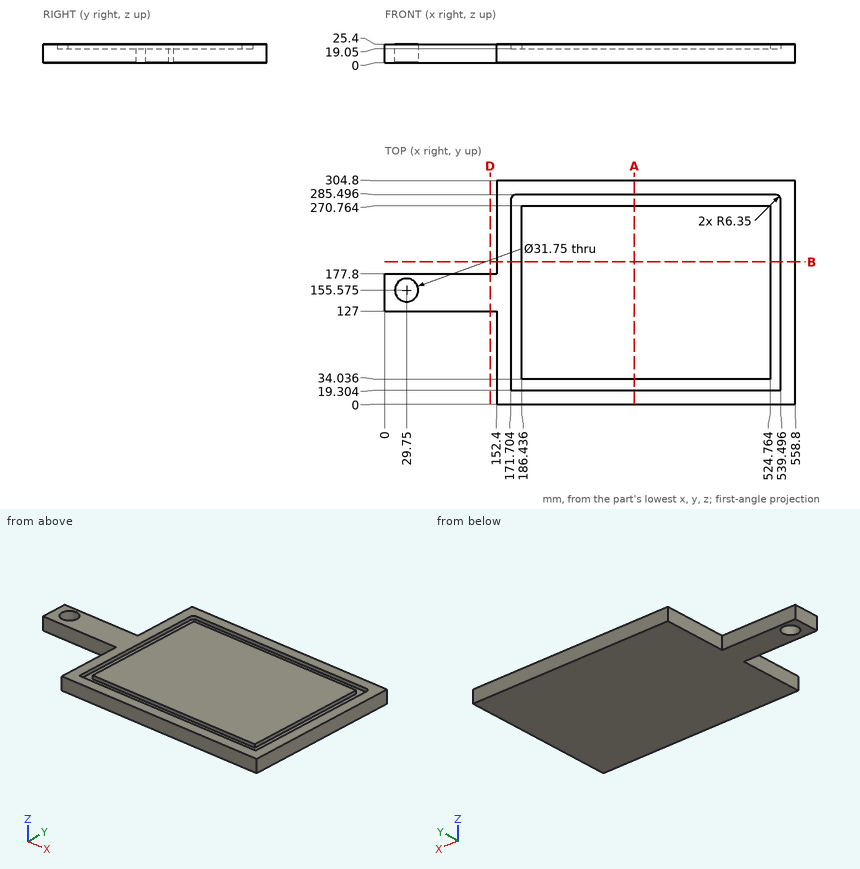
Geometry: see drawing. Coordinates: mm, zero at the bounding-box minimum. Coordinates: 2 decimals unless noted, no trailing zeros. Loops run counter-clockwise (first coordinate to the right, second up) from the corner with the lowest first, then second, coordinate; pieces in that order, holes last. Notation, with made-up numbers: (25.25, 65.5) - (76.25, 65.5) arc R26 cw to (76.25, 91.5) - close; hole circle Ø4 at (63, 47.25). An arc over 180 degrees is marked (long way). Return JSON: item names as keys, results as strings.
Q1. Section B-B, the plane y = 194. Return loops of the section in (x, z), plus the area to 3 significant figures.
Results:
{"outline": "(152.4, 0) - (558.8, 0) - (558.8, 25.4) - (539.5, 25.4) - (539.5, 19.05) - (524.76, 19.05) - (524.76, 25.4) - (186.44, 25.4) - (186.44, 19.05) - (171.7, 19.05) - (171.7, 25.4) - (152.4, 25.4) - close", "area": "10,100 mm2"}
Q2. Section A-A, the plane x = 340. Return loops of the section in (y, z).
Results:
{"outline": "(0, 0) - (304.8, 0) - (304.8, 25.4) - (285.5, 25.4) - (285.5, 19.05) - (270.76, 19.05) - (270.76, 25.4) - (34.04, 25.4) - (34.04, 19.05) - (19.3, 19.05) - (19.3, 25.4) - (0, 25.4) - close"}
Q3. Contact query for flat-ended pins moving along their axis: P1, Ø7.5, axis at x = 62.5, z = 14, coming from the +Y side; P2, Ø7.5, axis at x = 48, z = 17.5, coming from the -Y side; P3, Ø1.9, axis at y = 154, z = 23, coming from the -X side; P4, Ø19, axis at x = 29.75, y = 155.57, coming from the +Z side. Output: stop coordinate, or through.
Results:
{"P1": "y = 177.8", "P2": "y = 127", "P3": "x = 0", "P4": "through"}
Q4. Section D-D, the plane x = 143.5. Return loops of the section in (y, z).
Results:
{"outline": "(127, 0) - (177.8, 0) - (177.8, 25.4) - (127, 25.4) - close"}
Q5. Material intervals for line 1 along X through (y, z) = (50.5, 21.75); line 2 along X through (y, z) = (132, 24.25); line 3 along Y through (x, z) = (187.5, 19.5), sorted ascending.
Results:
{"line 1": "152.4 to 171.7, 186.44 to 524.76, 539.5 to 558.8", "line 2": "0 to 171.7, 186.44 to 524.76, 539.5 to 558.8", "line 3": "0 to 19.3, 34.04 to 270.76, 285.5 to 304.8"}
